Can you work these out from the model? Positions are in its coordinate system, mm. A direction names the side the tool comes from. Round coordinates to 2 decimals unless told otherwise and drop trailing zeros. Loops run counter-clockwise (first coordinate to the right, second up) from the corner with the lowest first, then second, coordinate; pieces in that order, holes last.
from build123d import *

# Parameters (mm, degrees)
F1_DEPTH = 50.8
F2_W     = 12.7
F2_H     = 25.4
F3_DEPTH = 25.4
F4_W     = 66.04
F4_H     = 20.32
F5_DEPTH = 3.81


# Not quite as in the source:
# - a feature names something its author has since deleted; it is built from what else it names


with BuildPart() as f1:
    # F0 (on Top) → F1 (new body)
    with BuildSketch(Plane.XY):
        Polygon((-3.3912816751, -25.752466172), (-69.4312816751, -25.752466172), (-36.4112816751, -38.452466172), align=None)
    extrude(amount=F1_DEPTH)

    # F2 (on face) → F3 (cut)
    with BuildSketch(Plane(origin=(0, -25.752466172, 0), x_dir=(-1, 0, 0), z_dir=(0, 1, 0))):
        with Locations((36.4112816751, 12.7)):
            Rectangle(F2_W, F2_H)
    extrude(amount=-F3_DEPTH, mode=Mode.SUBTRACT)

    # F4 (on face) → F5 (join)
    with BuildSketch(Plane(origin=(0, -25.752466172, 0), x_dir=(-1, 0, 0), z_dir=(0, 1, 0))):
        with Locations((36.4112816751, 40.64)):
            Rectangle(F4_W, F4_H)
    extrude(amount=F5_DEPTH)


solid = f1.part
(1) If we section it at D-D, the plane z = 32: List the corners of the cut face in (x, y) for me, then the cut area to 3 significant figures.
Worked answers:
outline: (-69.43, -25.75) - (-36.41, -38.45) - (-3.39, -25.75) - (-3.39, -21.94) - (-69.43, -21.94) - close
area: 671 mm2
(2) If we section it at C-C, the plane x = -27.5: List the corners of the cut face in (y, z) for me, then the cut area to 3 significant figures.
Worked answers:
outline: (-35.03, 0) - (-25.75, 0) - (-25.75, 30.48) - (-21.94, 30.48) - (-21.94, 50.8) - (-35.03, 50.8) - close
area: 548 mm2
(3) Will these pins go through, and if not, where does the flat tip stop? P1, Ø5, axis at x = -36.5, z = 27.5, coming from the +Y side; P2, Ø4, axis at x = -33.5, y = -34, coming from the -Z side; P3, Ø1.9, axis at x = -28, y = -24, coming from the -Z side.
Worked answers:
P1: stops at y = -25.75
P2: stops at z = 25.4
P3: stops at z = 30.48
(4) For faces 1 (the flat face through (-69.431, -24, 40)), 2 (the flat face through (-42.761, -31, 13)), 3 (the flat face through (-36, -24, 30.48)), which set-ups out of +Z, -Z, +X, -X, +Y, -Y let a thin tool reach every point of the face, with its end or its side?
Worked answers:
face 1: +Z, -Z, -X, +Y, -Y
face 2: -Z, +Y, -Y
face 3: -Z, +X, -X, +Y
(5) If I drill on line 1 (Z direction, x = -33, y = -24); line 2 (Y direction, x = -53.5, z = 34.5); line 3 (Y direction, x = -61, z = 16.5), over which ranges is the centre line in solid material (lowest first)?
Worked answers:
line 1: z = 30.48 to 50.8
line 2: y = -31.88 to -21.94
line 3: y = -29 to -25.75
(6) If we section it at A-A, the plane z = 13: List the corners of the cut face in (x, y) for me, then the cut area to 3 significant figures.
Worked answers:
outline: (-69.43, -25.75) - (-42.76, -36.01) - (-42.76, -25.75) - close; (-30.06, -36.01) - (-3.39, -25.75) - (-30.06, -25.75) - close
area: 274 mm2
(7) If we section it at B-B, the plane y = -32.5: List the corners of the cut face in (x, z) for me, then the cut area to 3 significant figures.
Worked answers:
outline: (-51.89, 0) - (-42.76, 0) - (-42.76, 25.4) - (-30.06, 25.4) - (-30.06, 0) - (-20.93, 0) - (-20.93, 50.8) - (-51.89, 50.8) - close
area: 1,250 mm2
(8) If we mould it in two halves opening along X, with no side actions, what happens to faces 4 (the flat face through (-3.391, -24, 40)), 5 (the flat face through (-36, -32, 25.4)), 6 (the flat face through (-36, -28, 50.8))? For each: released by +X, released by -X, zero draft, split by the parting line, or undercut.
Worked answers:
face 4: released by +X
face 5: undercut
face 6: zero draft
